from build123d import *

# Parameters (mm, degrees)
F0_W     = 7
F0_H     = 2
F1_DEPTH = 10
F0_W_2   = 4
F0_H_2   = 5
F0_H_3   = 3
F3_DEPTH = 6


with BuildPart() as f1:
    # F0 (on Front) → F1 (new body, symmetric)
    with BuildSketch(Plane.XZ):
        Polygon((-22.17742, -20), (17.82258, -20), (17.82258, 8), (17.82258, 10), (17.82258, 20), (9.82258, 20), (5.82258, 20), (-22.17742, 20), (-22.17742, 10), (-22.17742, 8), align=None)
        with Locations((-25.67742, 9)):
            Rectangle(F0_W, F0_H)
        with Locations((21.32258, 9)):
            Rectangle(F0_W, F0_H)
    extrude(amount=F1_DEPTH, both=True)

    # F0 (on Front) → F2 (revolve)
    with BuildSketch(Plane.XZ):
        with Locations((7.82258, 22.5)):
            Rectangle(F0_W_2, F0_H_2)
    revolve(axis=Axis((5.82258, 0, 22.5), (0, 0, 1)))

    # F0 (on Front) → F3 (join, symmetric)
    with BuildSketch(Plane.XZ):
        with Locations((3.82258, 26.5)):
            Rectangle(F0_W_2, F0_H_3)
        Polygon((5.82258, 25), (9.82258, 25), (40.82258, 25), (40.82258, 28), (5.82258, 28), align=None)
    extrude(amount=F3_DEPTH, both=True)


solid = f1.part
Input: part model. Units: mm. Frame: model coordinates. A direction names the side the tool comes from. Coordinates: 2 decimals unless noted, no trailing zeros. Write each loop counter-clockwise with the first axis right and the second up, starting at its lowest first coordinate (ties: lowest second). Pieces come first, ordered by that corner, then holes. Notation, with made-up numbers: M -16.5,36.25 L -6.5,36.25 A9 ccw -6.5,48.25 Z; hole C 22,64 d9. An arc over 180 degrees is marked long. Answer as a JSON object with one key per item and string values. Group by question number.
(1) Section C-C on x = -17.5. Output: boundary loops of the cut face in (y, z).
(2) Set-up query: faces 4 (the face through (17.823, 0, -6)), 5 (the face through (-22.177, 0, -6)), 6 (the face through (17.823, 0, 15)). Return all of +Z, -Z, +X, -X, +Y, -Y with unobstructed straight access to the full face (end or side cutting, diameter ignored); none if empty.
(3) Section B-B on y = 8.75. Output: boundary loops of the cut face in (x, z).
(4) Section A-A on x = 23. Output: boundary loops of the cut face in (y, z), plus the area to 3 significant figures.
(5) Contact query for flat-ended pins moving along their axis: P1, Ø12, axis at y = 5.5, z = -4.5, coming from the +X side; P2, Ø1.5, axis at x = 18, z = -11, coming from the -Y side; P3, Ø6, axis at x = 24.5, y = -1, coming from the -Z side; P4, Ø1.5, axis at x = 27, z = 26, coming from the -Y side. Output: stop coordinate, or through.
(6) Section D-D on z = -4. Output: boundary loops of the cut face in (x, y), plus the area to 3 significant figures.
(7) Ray query, line 1 along Z through (x, y) = (11, 2); line 2 along Z through (x, y) = (20, -2.5); line 3 along Z through (x, y) = (-4, -9). Return the intervals inside material, ascending. Write a range as [from, to].
(8) Mould query, pull axis Z, two halves, no side actions, for faces 1 (the face through (9.52, -1.53, 22.54)), 2 (the face through (-26, 0, 10)), 3 (the face through (21, 6, 27)). Classes: pulls with the +Z half, pulls with the -Z half, needs draft (parallel to the pull), parting line crosses it, or undercut.
Result set:
{
 "1": {"outline": "M -10,-20 L 10,-20 L 10,20 L -10,20 Z"},
 "2": {"face 4": "-Z, +X, +Y, -Y", "face 5": "-Z, -X, +Y, -Y", "face 6": "+X, +Y, -Y"},
 "3": {"outline": "M -29.18,8 L -22.18,8 L -22.18,-20 L 17.82,-20 L 17.82,8 L 24.82,8 L 24.82,10 L 17.82,10 L 17.82,20 L -22.18,20 L -22.18,10 L -29.18,10 Z"},
 "4": {"outline": "M -10,8 L 10,8 L 10,10 L -10,10 Z; M -6,25 L 6,25 L 6,28 L -6,28 Z", "area": "76.0 mm2"},
 "5": {"P1": "stops at x = 17.82", "P2": "stops at y = -10", "P3": "stops at z = 8", "P4": "stops at y = -6"},
 "6": {"outline": "M -22.18,-10 L 17.82,-10 L 17.82,10 L -22.18,10 Z", "area": "800 mm2"},
 "7": {"line 1": "z = [-20, 20], [25, 28]", "line 2": "z = [8, 10], [25, 28]", "line 3": "z = [-20, 20]"},
 "8": {"face 1": "undercut", "face 2": "pulls with the +Z half", "face 3": "needs draft"}
}
